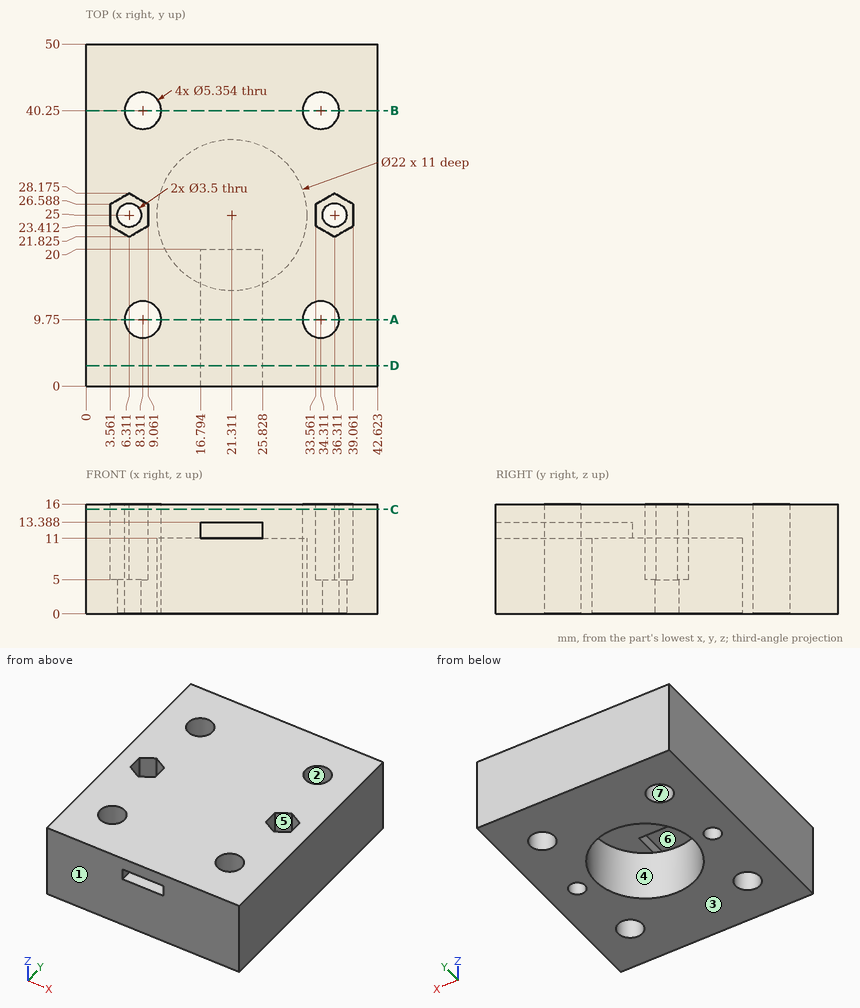
Drawing for the job (mm, zero at the part's lowest x, y, z). A direction names the side the tool comes from. Round coordinates to 2 decimals unless told otherwise and drop trailing zeros. Loops run counter-clockwise (first coordinate to the right, second up) from the corner with the lowest first, then second, coordinate; pieces in that order, holes last. Notation, with made-up numbers: (1, 63.5) -> (52, 63.5) arc R21 cw to (52, 77.5) -> close; hole circle Ø7 at (2, -21.75). An arc over 180 degrees is marked (long way). Use one line per item in the form item = value. Start each with the question number.
Item 1: Band-saw the part on D-D (y = 3). List the corners of the cut face in (x, z) (1 decimal).
Item 2: Drill centre lines: line 1 along X through (y, z) = (10, 8.75) (1 decimal); line 2 along X through (y, z) = (12.5, 12.75) (1 decimal); line 3 along Z through (x, y) = (11.5, 25.5). Where is each one in solid material? Low to high.
Item 3: Band-saw the part on C-C (z = 15.25). Give the number of separate pieces and of enclosed holes in the cut face, plus the area to 3 significant figures.
Item 4: Band-saw the part on A-A (y = 9.75). List the corners of the cut face in (x, z) (1 decimal).
Item 5: Two-plate mould, pull along Y, no slides. Class the marked faces 1, 2 and 3: released by +Y, released by -Y, zero draft, split by the parting line, or undercut.
Item 6: Band-saw the part on B-B (y = 40.25). List the corners of the cut face in (x, z) (1 decimal).
Item 7: Drop flat-ended pins along their axis: pin 1 Ø4.5 at (x, y) = (34.31, 40.25) entering from -Z; pin 2 Ø2 at (x, y) = (20.5, 16) entering from -Z; pin 3 Ø3 at (x, y) = (37.5, 24.5) entering from +Z. Give the stop position or say it passes through.
Item 8: Tool access for the marked faces 4, 5, 6 and 7: list every direction of +Z, -Z, +X, -X, +Y, -Y with a clear straight run to the whole face (end or side of a thin tool).
Data:
q1.outline = (0, 0) -> (42.6, 0) -> (42.6, 16) -> (0, 16) -> close; hole (16.8, 11) -> (25.8, 11) -> (25.8, 13.4) -> (16.8, 13.4) -> close
q2.line_1 = 0 to 5.6, 11 to 31.6, 37 to 42.6
q2.line_2 = 0 to 16.8, 25.8 to 42.6
q2.line_3 = 11 to 16
q3.separate_pieces = 1
q3.enclosed_holes = 6
q3.area = 1,990 mm^2
q4.outline = (0, 0) -> (5.6, 0) -> (5.6, 16) -> (0, 16) -> close; (11, 0) -> (31.6, 0) -> (31.6, 16) -> (11, 16) -> close; (37, 0) -> (42.6, 0) -> (42.6, 16) -> (37, 16) -> close; hole (16.8, 11) -> (25.8, 11) -> (25.8, 13.4) -> (16.8, 13.4) -> close
q5.face_1 = released by -Y
q5.face_2 = undercut
q5.face_3 = zero draft
q6.outline = (0, 0) -> (5.6, 0) -> (5.6, 16) -> (0, 16) -> close; (11, 0) -> (31.6, 0) -> (31.6, 16) -> (11, 16) -> close; (37, 0) -> (42.6, 0) -> (42.6, 16) -> (37, 16) -> close
q7.pin_1 = through
q7.pin_2 = 13.39
q7.pin_3 = 5
q8.face_4 = -Z
q8.face_5 = +Z
q8.face_6 = -Y
q8.face_7 = +Z, -Z
